CAD build for the part. Positions are in the model's coordinates, mm. A direction names the side the tool comes from. Give positions to 0.01 mm unless a question says otherwise; leave off trailing zeros. Order: outer loops, then holes, each group sorted by start corner. A loop starts at its lowest first (then second) coordinate and runs counter-clockwise, first axis right, second up.
Item 1: Wall check: L1, parallel to X at y = 7.25, z = -13; L2, parallel to X at y = 8, z = -23.5; L3, parallel to Z at x = 143, y = 10.25. Give the ranges that are in metal, low to high.
Item 2: Band-saw the part on B-B on x = 122. Give the cut face in (y, z).
Item 3: Two-plate mould, pull along X, no slides. Class faces 1 (the flat face through (190, 13, -7.5)), 2 (the cylindrical face through (166, 12.54, -23.57)), 3 (the flat face through (0, 6, -15)): released by +X, released by -X, zero draft, split by the parting line, or undercut.
Item 4: Which spindle directions (+Z, -Z, +X, -X, +Y, -Y) get a long thin tool onto all of the face, cutting with end or side? Do faces 4 (the flat face through (98.6, 15, -25.2)), 5 (the flat face through (10, 13, -22.5)), 6 (the flat face through (32.5, 13, -15)), 7 (the flat face through (186, 10, -15)), 8 (the flat face through (99, 7, -30)). Say none if no direction does.
Item 5: Band-saw the part on A-A on z = -15. Give the cut face in (x, y).
Item 6: Flat gauge pins, fed straight in: P1, Ø4, axis at y = 13.5, z = -16.5, coming from the -X side; P2, Ø1.5, axis at x = 161, z = -18, coming from the +Y side. Where does each tip first touch, or does it go through?
Item 7: Band-saw the part on C-C on x = 35. Give the cut face in (y, z), plus the area to 3 significant figures.
```python
from build123d import *

# Parameters (mm, degrees)
SKETCH1_W           = 200
SKETCH1_H           = 30
BOSS_EXTRUDE1_DEPTH = 15
CUT_EXTRUDE1_DEPTH  = 5
SKETCH3_R           = 0.75
CUT_EXTRUDE2_DEPTH  = 30
CUT_EXTRUDE3_DEPTH  = 5


with BuildPart() as part:
    # Sketch1 → Boss-Extrude1 (new body)
    with BuildSketch(Plane(origin=(0, 0, 0), x_dir=(1, 0, 0), z_dir=(0, 1, 0))):
        with Locations((100, 15)):
            Rectangle(SKETCH1_W, SKETCH1_H)
    extrude(amount=BOSS_EXTRUDE1_DEPTH)

    # Sketch2 → Cut-Extrude1 (cut)
    with BuildSketch(Plane(origin=(0, 15, 0), x_dir=(1, 0, 0), z_dir=(0, 1, 0))):
        with BuildLine():
            Line((-20, 22.5), (20, 22.5))
            ThreePointArc((20, 22.5), (27.5, 15), (20, 7.5))
            Line((20, 7.5), (-20, 7.5))
            ThreePointArc((-20, 7.5), (-27.5, 15), (-20, 22.5))
        make_face()
        with BuildLine():
            Line((220, 22.5), (180, 22.5))
            ThreePointArc((180, 22.5), (172.5, 15), (180, 7.5))
            Line((180, 7.5), (220, 7.5))
            ThreePointArc((220, 7.5), (227.5, 15), (220, 22.5))
        make_face()
    extrude(amount=-CUT_EXTRUDE1_DEPTH, mode=Mode.SUBTRACT)

    # Sketch3 → Cut-Extrude2 (cut)
    with BuildSketch(Plane.XY):
        with Locations((25, 7.5)):
            Circle(SKETCH3_R)
        with Locations((75, 7.5)):
            Circle(SKETCH3_R)
        with Locations((125, 7.5)):
            Circle(SKETCH3_R)
        with Locations((175, 7.5)):
            Circle(SKETCH3_R)
    extrude(amount=-CUT_EXTRUDE2_DEPTH, mode=Mode.SUBTRACT)

    # Sketch4 → Cut-Extrude3 (cut)
    with BuildSketch(Plane(origin=(0, 15, 0), x_dir=(1, 0, 0), z_dir=(0, 1, 0))):
        with BuildLine():
            Line((37.5, 25), (162.5, 25))
            ThreePointArc((162.5, 25), (166.035533906, 23.535533906), (167.5, 20))
            Line((167.5, 20), (167.5, 10))
            ThreePointArc((167.5, 10), (166.035533906, 6.464466094), (162.5, 5))
            Line((162.5, 5), (37.5, 5))
            ThreePointArc((37.5, 5), (33.964466094, 6.464466094), (32.5, 10))
            Line((32.5, 10), (32.5, 20))
            ThreePointArc((32.5, 20), (33.964466094, 23.535533906), (37.5, 25))
        make_face()
    extrude(amount=-CUT_EXTRUDE3_DEPTH, mode=Mode.SUBTRACT)


solid = part.part
```
The answers:
1. L1: x = 0 to 24.29, 25.71 to 74.29, 75.71 to 124.29, 125.71 to 174.29, 175.71 to 200
1. L2: x = 0 to 24.44, 25.56 to 74.44, 75.56 to 124.44, 125.56 to 174.44, 175.56 to 200
1. L3: z = -30 to -25, -5 to 0
2. outline: (0, -30) - (15, -30) - (15, -25) - (10, -25) - (10, -5) - (15, -5) - (15, 0) - (0, 0) - close
3. face 1: zero draft
3. face 2: undercut
3. face 3: released by -X
4. face 4: +Z, -Z, +X, -X, +Y
4. face 5: -X, +Y
4. face 6: +Y
4. face 7: +X, +Y
4. face 8: -Z, +X, -X, +Y, -Y
5. outline: (0, 0) - (200, 0) - (200, 10) - (172.5, 10) - (172.5, 15) - (167.5, 15) - (167.5, 10) - (32.5, 10) - (32.5, 15) - (27.5, 15) - (27.5, 10) - (0, 10) - close; hole circle Ø1.5 at (25, 7.5); hole circle Ø1.5 at (75, 7.5); hole circle Ø1.5 at (125, 7.5); hole circle Ø1.5 at (175, 7.5)
6. P1: stops at x = 26.63
6. P2: stops at y = 10
7. outline: (0, -30) - (15, -30) - (15, -24.33) - (10, -24.33) - (10, -5.67) - (15, -5.67) - (15, 0) - (0, 0) - close
7. area: 357 mm2
